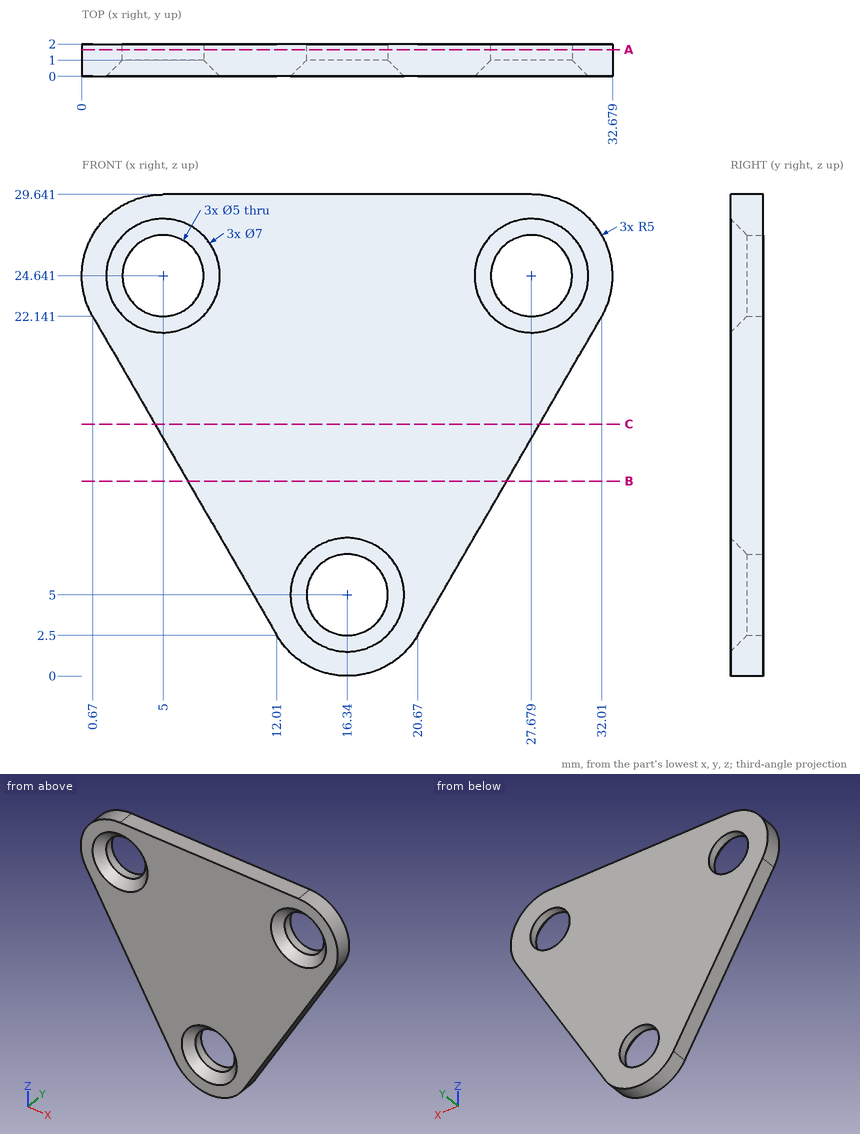
Part print with two shaded views. Sizes in mm from the minimum x, y, z corner. Coordinates: 2 decimals unless noted, no trailing zeros. Write each loop counter-clockwise with the first axis right and the second up, starting at its lowest first coordinate (ties: lowest second). Pieces come first, ordered by that corner, then holes. Notation, with made-up numbers: (17, 58) - (50, 58) arc R20 cw to (50, 71) - close; hole circle Ø11 at (24, 32.25). An arc over 180 degrees is marked (long way). Use a Markdown table: item, result. Add a question column.
Item 1: Band-saw the part on C-C, the plane z = 15.5. Write the cut outline in (x, y) (1 decimal).
Item 2: Band-saw the part on A-A, the plane y = 1.65. Write the cut outline in (x, z).
Item 3: Drill centre lines: line 1 along X through (y, z) = (1.25, 22.5) (1 decimal); line 2 along Z through (x, y) = (5, 1.5) (1 decimal); line 3 along Z through (x, y) = (4.5, 0.5) (1 decimal). Where is each one in solid material? Low to high.
Item 4: Band-saw the part on B-B, the plane z = 12. Write the cut outline in (x, y) (1 decimal).
Item 5: Drop a flat-ended pin along its axis: pin 1 (6 mm diameter, centred on x = 5, z = 24.64, fed in from +Y). Give the stop position or say it passes through.
A:
| question | item | result |
|---|---|---|
| 1 | outline | (4.5, 0) - (28.2, 0) - (28.2, 2) - (4.5, 2) - close |
| 2 | outline | (0.67, 22.14) - (12.01, 2.5) arc R5 ccw to (20.67, 2.5) - (32.01, 22.14) arc R5 ccw to (27.68, 29.64) - (5, 29.64) arc R5 ccw to start; hole circle Ø5 at (5, 24.64); hole circle Ø5 at (16.34, 5); hole circle Ø5 at (27.68, 24.64) |
| 3 | line 1 | x = 0.5 to 3.7, 6.3 to 26.4, 29 to 32.2 |
| 3 | line 2 | z = 14.6 to 22.1, 27.1 to 29.6 |
| 3 | line 3 | z = 15.5 to 21.7, 27.6 to 29.6 |
| 4 | outline | (6.5, 0) - (26.2, 0) - (26.2, 2) - (6.5, 2) - close |
| 5 | pin 1 | stops at y = 2 |
